The listing builds one solid part. Answer for the finished solid, in the listing's coordinates (mm). A direction names the side the tool comes from. Coordinates: 2 decimals unless noted, no trailing zeros. Order: outer loops, then holes, each group sorted by start corner. A loop starts at its lowest first (then second) coordinate and runs counter-clockwise, first axis right, second up. Notation, with made-up numbers: (16, 79.5) - (53, 79.5) arc R24 ccw to (53, 105.5) - close; hole circle Ø7 at (-7.5, -20.75). An arc over 180 degrees is marked (long way). Use one line per item in the form item = value. Start each with the question number.
Item 1: A tool of negligible diameter and unlimited length cuts with its end or side. For faces 5 (the flat face through (58.3, -60, -6)), 6 (the flat face through (14, -65, -6.6)), 7 (the flat face through (-13, -35.6, -7)), from which of +Z, -Z, +X, -X, +Y, -Y can it reach the whole face along a straight path? Write none if from no direction.
Item 2: Section A-A, the plane x = 12.7 is taken. Write down the section's boundary in (y, z).
Item 3: Each of these flat-tipped pins is pushed along its axis until it touches: pin 1 Ø2.5 at (x, y) = (28.5, -16.5) entering from +Z; pin 2 Ø4 at (x, z) = (36, -4.5) entering from +Y; pin 3 Ø1 at (x, z) = (-10, -4.5) entering from -Y (3 decimals); pin 4 Ø3.5 at (y, z) = (-50.5, -6) entering from -X. Where does it stop, or does it pass through?
Item 4: Section B-B, the plane y = -50.9 is taken. Write down the section's boundary in (x, z).
Item 5: Consider line 1 along X through (y, z) = (-60, -8); line 2 along Y through (x, z) = (29, -7.25); line 3 along X through (y, z) = (-19.5, -7.5). Determine where each line is inside the solid, lowest interval first. Write a range as [from, to].
Item 6: Section D-D, the plane y = -25.1 is taken. Write down the section's boundary in (x, z).
Item 7: The mould has two halves that part along X. Classify faces 1 (the cylindrical face through (-0.16, -49.71, -4.21)), 2 (the flat face through (-45, -46.6, -5)), 3 (the flat face through (11.7, -36.8, -5.2)), 4 (the flat face through (-14.9, -38, -7)): released by +X, released by -X, zero draft, split by the parting line, or undercut.
Item 8: Section C-C, the plane x = 0 is taken. Write down the section's boundary in (y, z).
from build123d import *

# Parameters (mm, degrees)
PAD010_DEPTH  = 1.6
SKETCH055_W   = 15.4
SKETCH055_H   = 12
SKETCH055_W_2 = 15
SKETCH055_H_2 = 23.5
SKETCH055_W_3 = 34
SKETCH055_H_3 = 25.4
PAD011_DEPTH  = 1.6
SKETCH056_W   = 26
SKETCH056_H   = 26
PAD012_DEPTH  = 5.8
SKETCH057_W   = 20
SKETCH057_H   = 14
PAD013_DEPTH  = 4
SKETCH058_W   = 12.4
SKETCH058_H   = 8
PAD014_DEPTH  = 5
SKETCH059_W   = 7.4
SKETCH059_H   = 9
PAD015_DEPTH  = 3
SKETCH060_W   = 4.4
SKETCH060_H   = 4.4
PAD016_DEPTH  = 3
SKETCH061_R   = 1.2
PAD017_DEPTH  = 2


with BuildPart() as part:
    # Sketch053 → Pad010 (new body)
    with BuildSketch(Plane.XY):
        with BuildLine():
            Line((-59.3, -6.6), (-3.2, -6.6))
            Line((-3.2, -6.6), (-3.2, -11.6))
            ThreePointArc((-3.2, -11.6), (0, -14.8), (3.2, -11.6))
            Line((3.2, -6.6), (3.2, -11.6))
            Line((3.2, -6.6), (59.3, -6.6))
            Line((59.3, -6.6), (59.3, -36.9))
            Line((59.3, -36.9), (54.3, -36.9))
            ThreePointArc((54.3, -36.9), (51.1, -40.1), (54.3, -43.3))
            Line((59.3, -43.3), (54.3, -43.3))
            Line((59.3, -43.3), (59.3, -73.6))
            Line((59.3, -73.6), (3.2, -73.6))
            Line((3.2, -73.6), (3.2, -68.6))
            ThreePointArc((3.2, -68.6), (0, -65.4), (-3.2, -68.6))
            Line((-3.2, -73.6), (-3.2, -68.6))
            Line((-3.2, -73.6), (-59.3, -73.6))
            Line((-59.3, -73.6), (-59.3, -43.3))
            Line((-59.3, -43.3), (-54.3, -43.3))
            ThreePointArc((-54.3, -43.3), (-51.1, -40.1), (-54.3, -36.9))
            Line((-59.3, -36.9), (-54.3, -36.9))
            Line((-59.3, -36.9), (-59.3, -6.6))
        make_face()
    extrude(amount=PAD010_DEPTH)

    # Sketch055 (on Face22 of Pad010) → Pad011 (join)
    with BuildSketch(Plane.XY.offset(1.6)):
        with Locations((14.6, -65.2)):
            Rectangle(SKETCH055_W, SKETCH055_H)
        with Locations((51.4, -20.25)):
            Rectangle(SKETCH055_W_2, SKETCH055_H_2)
        with Locations((41.3, -59.9)):
            Rectangle(SKETCH055_W_3, SKETCH055_H_3)
    extrude(amount=PAD011_DEPTH)

    # Sketch056 (on Face5 of Pad011) → Pad012 (join)
    with BuildSketch(Plane.XY.offset(1.6)):
        with Locations((-45.1, -59.6)):
            Rectangle(SKETCH056_W, SKETCH056_H)
    extrude(amount=PAD012_DEPTH)

    # Sketch057 (on Face5 of Pad012) → Pad013 (join)
    with BuildSketch(Plane.XY.offset(1.6)):
        with Locations((-46.3, -16.4)):
            Rectangle(SKETCH057_W, SKETCH057_H)
    extrude(amount=PAD013_DEPTH)

    # Sketch058 (on Face5 of Pad013) → Pad014 (join)
    with BuildSketch(Plane.XY.offset(1.6)):
        with Locations((28.1, -14.6)):
            Rectangle(SKETCH058_W, SKETCH058_H)
    extrude(amount=PAD014_DEPTH)

    # Sketch059 (on Face47 of Pad014) → Pad015 (join)
    with BuildSketch(Plane.XY.offset(3.2)):
        with Locations((54.6, -59.7)):
            Rectangle(SKETCH059_W, SKETCH059_H)
    extrude(amount=PAD015_DEPTH)

    # Sketch060 (on Face5 of Pad015) → Pad016 (join)
    with BuildSketch(Plane.XY.offset(1.6)):
        with Locations((-12.7, -37.8)):
            Rectangle(SKETCH060_W, SKETCH060_H)
        with Locations((0, -25.1)):
            Rectangle(SKETCH060_W, SKETCH060_H)
        with Locations((12.7, -37.8)):
            Rectangle(SKETCH060_W, SKETCH060_H)
        with Locations((0, -50.9)):
            Rectangle(SKETCH060_W, SKETCH060_H)
    extrude(amount=PAD016_DEPTH)

    # Sketch061 (on Face71 of Pad016) → Pad017 (join)
    with BuildSketch(Plane.XY.offset(4.6)):
        with Locations((-12.7, -37.8)):
            Circle(SKETCH061_R)
        with Locations((0, -25.1)):
            Circle(SKETCH061_R)
        with Locations((12.7, -37.8)):
            Circle(SKETCH061_R)
        with Locations((0, -50.9)):
            Circle(SKETCH061_R)
    extrude(amount=PAD017_DEPTH)


with BuildPart() as part_1:
    # Body008 placement: moved
    add(part.part.moved(Location((0, 0, -9.8))))


solid = part_1.part
Response:
q1.face_5 = +Z, +X, -Y
q1.face_6 = +Z, -Y
q1.face_7 = +Z, +X, -X, +Y
q2.outline = (-73.6, -9.8) - (-6.6, -9.8) - (-6.6, -8.2) - (-35.6, -8.2) - (-35.6, -5.2) - (-36.6, -5.2) - (-36.6, -3.2) - (-39, -3.2) - (-39, -5.2) - (-40, -5.2) - (-40, -8.2) - (-59.2, -8.2) - (-59.2, -6.6) - (-71.2, -6.6) - (-71.2, -8.2) - (-73.6, -8.2) - close
q3.pin_1 = -3.2
q3.pin_2 = -10.6
q3.pin_3 = through
q3.pin_4 = -58.1
q4.outline = (-59.3, -9.8) - (59.3, -9.8) - (59.3, -8.2) - (58.3, -8.2) - (58.3, -6.6) - (24.3, -6.6) - (24.3, -8.2) - (2.2, -8.2) - (2.2, -5.2) - (1.2, -5.2) - (1.2, -3.2) - (-1.2, -3.2) - (-1.2, -5.2) - (-2.2, -5.2) - (-2.2, -8.2) - (-32.1, -8.2) - (-32.1, -2.4) - (-58.1, -2.4) - (-58.1, -8.2) - (-59.3, -8.2) - close
q5.line_1 = [-58.1, -32.1], [6.9, 22.3], [24.3, 58.3]
q5.line_2 = [-72.6, -47.2], [-18.6, -10.6]
q5.line_3 = [-56.3, -36.3], [43.9, 58.9]
q6.outline = (-59.3, -9.8) - (59.3, -9.8) - (59.3, -8.2) - (58.9, -8.2) - (58.9, -6.6) - (43.9, -6.6) - (43.9, -8.2) - (2.2, -8.2) - (2.2, -5.2) - (1.2, -5.2) - (1.2, -3.2) - (-1.2, -3.2) - (-1.2, -5.2) - (-2.2, -5.2) - (-2.2, -8.2) - (-59.3, -8.2) - close
q7.face_1 = undercut
q7.face_2 = zero draft
q7.face_3 = undercut
q7.face_4 = released by -X
q8.outline = (-65.4, -9.8) - (-14.8, -9.8) - (-14.8, -8.2) - (-22.9, -8.2) - (-22.9, -5.2) - (-23.9, -5.2) - (-23.9, -3.2) - (-26.3, -3.2) - (-26.3, -5.2) - (-27.3, -5.2) - (-27.3, -8.2) - (-48.7, -8.2) - (-48.7, -5.2) - (-49.7, -5.2) - (-49.7, -3.2) - (-52.1, -3.2) - (-52.1, -5.2) - (-53.1, -5.2) - (-53.1, -8.2) - (-65.4, -8.2) - close
